Answer from the drawing. Dimensions are ordinates in mm from the lowest x, y and z of the part. Coordinates: 2 decimals unless noted, no trailing zeros. Write each loop counter-clockwise with the first axis right and the second up, starting at its lowest first coordinate (ties: lowest second). Pieces come first, ordered by that corner, then holes.
(1) The part is cut by section D-D, the plane y = 2.15. Determine the outline of the cut face in (x, z) (3 decimals).
(2) The part is cut by section A-A, the plane z = 6.25. Determine the outline of the cut face in (x, y).
(3) Given pin 1 (7.5 mm diameter, centred on x = 6.25, z = 6.25, fed in from -Y); pin 2 (1 mm diameter, centred on x = 11, y = 1, fed in from -Z); pin 3 (3 mm diameter, centred on x = 6.5, z = 3, fed in from +Y), each flat-ended and moving along its own axis, determine where each tip first touches the part or whether it passes through.
(4) Straight lines are drawn through the part: line 1 along Z through (x, y) = (6.25, 1.65); line 2 along Z through (x, y) = (3.5, 0.85); line 3 along X through (y, z) = (2.6, 7.5). For each, find the intervals that lie inside material, in ascending order.
(5) The part is cut by section B-B, the plane x = 6.25. Determine the outline of the cut face in (y, z).
(6) Determine the mould class of the marked faces 1, 2 and 3 for opening direction X: pulls with the +X half, pulls with the -X half, needs draft (parallel to the pull), parting line crosses it, or undercut.
(7) The part is cut by section C-C, the plane y = 1.45. Determine the outline of the cut face in (x, z), and give its area (3 significant figures).
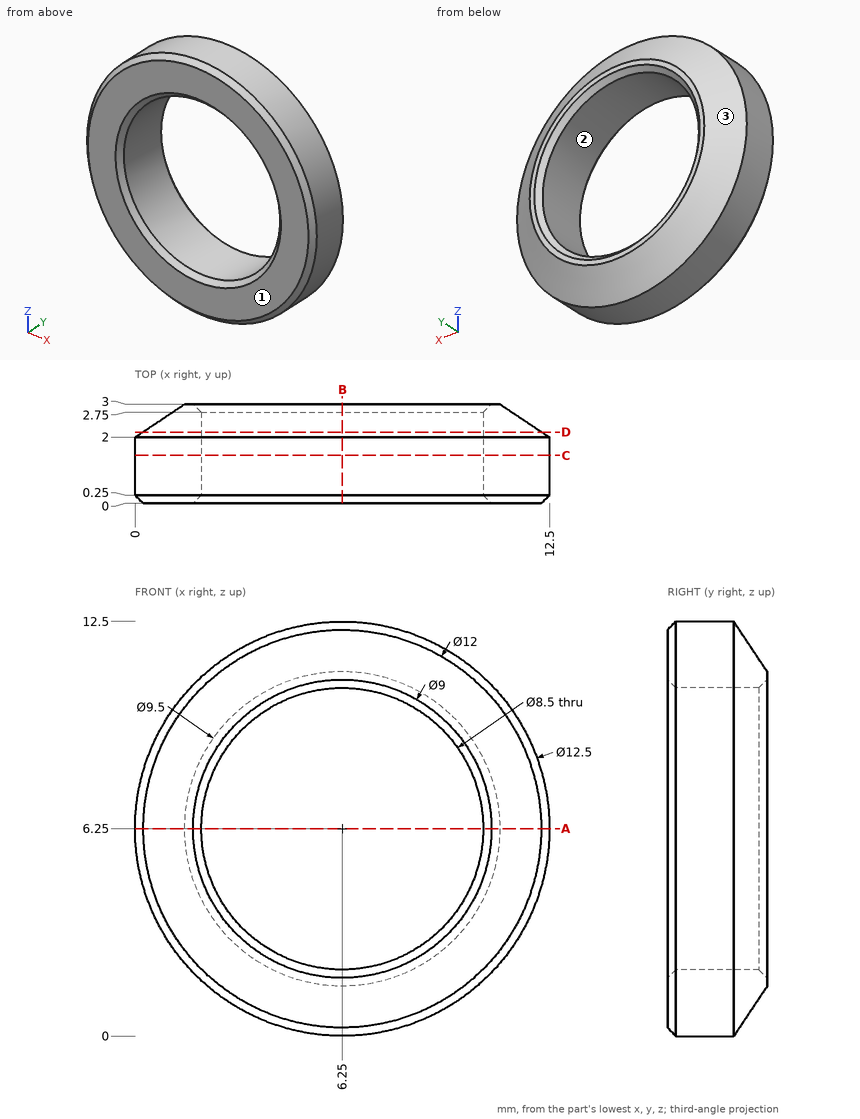
Computed:
1. outline: circle Ø12.05 at (6.25, 6.25); hole circle Ø8.5 at (6.25, 6.25)
2. outline: (0, 0.25) - (0.25, 0) - (1.75, 0) - (2, 0.25) - (2, 2.75) - (1.75, 3) - (1.5, 3) - (0, 2) - close; (10.5, 0.25) - (10.75, 0) - (12.25, 0) - (12.5, 0.25) - (12.5, 2) - (11, 3) - (10.75, 3) - (10.5, 2.75) - close
3. pin 1: passes through
3. pin 2: stops at z = 1.67
3. pin 3: stops at y = 3
4. line 1: z = 0 to 2, 10.5 to 12.5
4. line 2: z = 0.64 to 3.01, 9.49 to 11.86
4. line 3: x = 1.05 to 2.19, 10.31 to 11.45
5. outline: (0, 0.25) - (0.25, 0) - (2, 0) - (3, 1.5) - (3, 1.75) - (2.75, 2) - (0.25, 2) - (0, 1.75) - close; (0, 10.75) - (0.25, 10.5) - (2.75, 10.5) - (3, 10.75) - (3, 11) - (2, 12.5) - (0.25, 12.5) - (0, 12.25) - close
6. face 1: needs draft
6. face 2: undercut
6. face 3: parting line crosses it
7. outline: circle Ø12.5 at (6.25, 6.25); hole circle Ø8.5 at (6.25, 6.25)
7. area: 66.0 mm2
